from build123d import *

# Parameters (mm, degrees)
F1_DEPTH = 6.35
F3_DEPTH = 25.4
F4_R     = 3.81


with BuildPart() as f1:
    # F0 (on Top) → F1 (new body, symmetric)
    with BuildSketch(Plane.XY):
        with BuildLine():
            Line((-63.5, 0), (63.5, 0))
            ThreePointArc((63.5, 0), (0, 63.5), (-63.5, 0))
        make_face()
    extrude(amount=F1_DEPTH, both=True)

    # F2 (on Top) → F3 (cut)
    with BuildSketch(Plane.XY):
        with BuildLine():
            Line((-50.2836502119, 7.2245775906), (50.2836502119, 7.2245775906))
            ThreePointArc((50.2836502119, 7.2245775906), (0, 50.8), (-50.2836502119, 7.2245775906))
        make_face()
    extrude(amount=-F3_DEPTH, mode=Mode.SUBTRACT)

    # F6: sweep along a path in F5
    with BuildLine(Plane.YZ) as f6_path:
        Line((25.5370624363, 0), (6.1716223136, -26.4036767185))
    # F4 (on Top) → F6 (sweep)
    with BuildSketch(Plane.XY):
        with Locations((0, 25.4)):
            Circle(F4_R)
    sweep(path=f6_path.line)


solid = f1.part
Verification items for the finished model (mm, model axes). A direction names the side the tool comes from. Round coordinates to 2 decimals unless told otherwise and drop trailing zeros. Write each loop counter-clockwise with the first axis right and the second up, starting at its lowest first coordinate (ties: lowest second). Pieces come first, ordered by that corner, then holes.
(1) Section check C-C (z = -2.5). Give the number of separate pieces and of enclosed holes in the cut face, plus the area to 3 significant figures.
Returned:
separate pieces: 2
enclosed holes: 1
area: 3,060 mm2
(2) Mould release check, pull along X, two halves, no side actions. Record for faces 3 (the cylindrical face through (1.396, 63.485, 0.089)), 4 (the flat face through (-0.7, 29.3, 0)), 5 (the flat face through (-1, 53, -6.35)): pulls with the +X half, pulls with the -X half, needs draft (parallel to the pull), parting line crosses it, or undercut.
Returned:
face 3: parting line crosses it
face 4: undercut
face 5: needs draft
(3) Section check D-D (y = 58.5). Enter the section's corners in (x, z).
Returned:
outline: (-24.7, -6.35) - (24.7, -6.35) - (24.7, 6.35) - (-24.7, 6.35) - close
(4) Depth check by flat-ended pin: pin 1 Ø3 at (x, y) = (-32, 14.5) entering from -Z; pin 2 Ø3 at (y, z) = (32.5, -4) entering from +X; pin 3 Ø10 at (x, y) = (-8.5, 54) entering from -Z. Enter the tip coordinate at first touch or a pass-through.
Returned:
pin 1: stops at z = 0
pin 2: stops at x = 55.42
pin 3: stops at z = -6.35
(5) Access from +Z, -Z, +X, -X, +Y, -Y to the whole of each face (thin tool, end or side, straight path). Record for faces 1 (the flat face through (-1, 0, 0)), 2 (the cylindrical face through (1.02, 50.79, -3.13)).
Returned:
face 1: +Z, -Z, +X, -X, -Y
face 2: -Z
(6) Section check B-B (y = 41). Enter the section's corners in (x, z).
Returned:
outline: (-48.49, -6.35) - (-29.99, -6.35) - (-29.99, 0) - (29.99, 0) - (29.99, -6.35) - (48.49, -6.35) - (48.49, 6.35) - (-48.49, 6.35) - close
(7) Section check A-A (x = -23). Enter the section's corners in (y, z).
Returned:
outline: (0, -6.35) - (7.22, -6.35) - (7.22, 0) - (45.3, 0) - (45.3, -6.35) - (59.19, -6.35) - (59.19, 6.35) - (0, 6.35) - close
(8) Material ranges on line 1 (Z direction, x = -24.5, y = 19.5); line 2 (Z direction, x = 47.5, y = 34); line 3 (X direction, y = 28, z = -3.5), recorded low to high.
Returned:
line 1: z = 0 to 6.35
line 2: z = -6.35 to 6.35
line 3: x = -56.99 to -42.39, 42.39 to 56.99
